CAD build for the part. Positions are in the model's coordinates, mm. Coordinates: 2 decimals unless noted, no trailing zeros. Write each loop counter-clockwise with the first axis right and the second up, starting at its lowest first coordinate (ties: lowest second). Pieces come first, ordered by that corner, then holes. Notation, with made-up numbers: (79.5, 58.25) - (121.5, 58.25) arc R4 cw to (121.5, 64.25) - close; hole circle Ø11 at (-28, 26). An arc over 180 degrees is marked (long way). One line per question, with ' | ' between items. Start each with the question number.
1. Probe line 1 (X direction, y = 2.5, z = 1.5); line 2 (Y direction, x = 70.5, z = 1.35); line 3 (X direction, y = 4.5, z = 1.45). List the from-to ranges inside material, lowest first.
2. Band-saw the part on A-A, the plane y = 14.5. Write the cut outline in (x, z), then the cut area to 3 significant figures.
3. Flat gauge pins, fed straight in: P1, Ø8, axis at x = 46, y = 10.5, coming from the -Z side; P2, Ø0.6, axis at y = 0.5, z = 0.5, coming from the +X side. Where does each tip first touch, or does it go through?
from build123d import *

# Parameters (mm, degrees)
EXTRUDE_1_DEPTH = 2
FILLET_1_R      = 2


with BuildPart() as part:
    # 草图1 → 凸台-拉伸1 (new body)
    with BuildSketch(Plane.XY):
        Polygon((81.543574606, -5.900283983), (76.543576359, -5.904470333), (76.543576359, 3.08), (72.531874134, 3.08), (72.531874134, 1.58), (69.331874134, 1.58), (69.331874134, 3.08), (66.131874134, 3.08), (66.131874134, 7.08), (69.331874134, 7.08), (69.331874134, 8.58), (72.531874134, 8.58), (72.531874134, 7.08), (76.531874134, 7.08), (76.520862712, 16.085955117), (81.520858939, 16.092097641), (81.533074683, 24.092088314), (76.533079924, 24.099327787), (-95.466920076, 24.099327787), (-100.466914835, 24.092088314), (-100.454699091, 16.092097641), (-95.454702864, 16.085955117), (-95.465714286, 7.08), (-91.465714286, 7.08), (-91.465714286, 8.58), (-88.265714286, 8.58), (-88.265714286, 7.08), (-85.065714286, 7.08), (-85.065714286, 3.08), (-88.265714286, 3.08), (-88.265714286, 1.58), (-91.465714286, 1.58), (-91.465714286, 3.08), (-95.47741651, 3.08), (-95.47741651, -5.904470333), (-100.477414758, -5.900283983), (-100.506156647, -13.900232352), (-95.506187511, -13.917800667), (76.57234736, -13.917800667), (81.572316495, -13.900232352), align=None)
    extrude(amount=EXTRUDE_1_DEPTH)

    # 圆角1
    fillet_1_edges = [part.edges().sort_by_distance(p)[0] for p in [
        (-100.506156647, -13.900232352, 1),
        (-100.477414758, -5.900283983, 1),
        (-100.454699091, 16.092097641, 1),
        (-100.466914835, 24.092088314, 1),
        (81.533074683, 24.092088314, 1),
        (81.520858939, 16.092097641, 1),
        (81.543574606, -5.900283983, 1),
        (81.572316495, -13.900232352, 1),
    ]]
    fillet(fillet_1_edges, radius=FILLET_1_R)


solid = part.part
Filled in:
1) line 1: x = -95.48 to -91.47, -88.27 to 69.33, 72.53 to 76.54 | line 2: y = -13.92 to 1.58, 8.58 to 24.1 | line 3: x = -85.07 to 66.13
2) outline: (-95.46, 0) - (76.52, 0) - (76.52, 2) - (-95.46, 2) - close | area: 344 mm²
3) P1: stops at z = 0 | P2: stops at x = 76.54
